Read the model definition and answer for the solid it produces. Units are mm, in the model's axes. A direction names the side the tool comes from. Coordinates: 2 decimals unless noted, no trailing zeros. Order: outer loops, then holes, each group sorted by start corner. A loop starts at its lowest first (then second) coordinate and runs counter-clockwise, first axis right, second up.
```python
from build123d import *

# Parameters (mm, degrees)
SKETCH1_W                   = 3
SKETCH1_H                   = 96
BOSS_EXTRUDE1_DEPTH         = 44.45
SKETCH2_W                   = 20
SKETCH2_H                   = 16
SKETCH2_R                   = 4
BOSS_EXTRUDE2_DEPTH         = 4
FILLET2_RADIUS              = 8
FILLET2_LENGTH              = 4
FILLET2_OF_MIRROR2_2_RADIUS = 8
FILLET2_OF_MIRROR2_2_LENGTH = 4


with BuildPart() as part:
    # Sketch1 → Boss-Extrude1 (new body)
    with BuildSketch(Plane.XY):
        Rectangle(SKETCH1_W, SKETCH1_H)
    extrude(amount=BOSS_EXTRUDE1_DEPTH)

    # Sketch2 → Boss-Extrude2 (add)
    with BuildSketch(Plane.XY.offset(44.45)):
        with Locations((11.5, -40)):
            Rectangle(SKETCH2_W, SKETCH2_H)
        with Locations((15.5, -40)):
            Circle(SKETCH2_R, mode=Mode.SUBTRACT)
    boss_extrude2 = extrude(amount=-BOSS_EXTRUDE2_DEPTH)

    # Fillet2: full round fillet: the end face becomes a half cylinder, R = half its width
    fillet2_face = Plane((21.5, -40, 42.45), x_dir=(0, 0, -1), z_dir=(1, 0, 0))  # on the end face: x along it, z out of the body
    fillet2_slab = fillet2_face.offset(-FILLET2_RADIUS / 2) * Box(FILLET2_LENGTH, 2 * FILLET2_RADIUS, FILLET2_RADIUS, mode=Mode.PRIVATE)  # the body's end, R deep
    fillet2_round = Plane((13.5, -40, 42.45), x_dir=(1, 0, 0), z_dir=(0, 0, -1)) * Cylinder(FILLET2_RADIUS, FILLET2_LENGTH, mode=Mode.PRIVATE)  # its axis R under the face
    add(fillet2_slab - fillet2_round, mode=Mode.SUBTRACT)

    # Mirror2: Boss-Extrude2 across plane
    add(boss_extrude2.mirror(Plane.XY.offset(22.225)))

    # Fillet2 of Mirror2 2: full round fillet: the end face becomes a half cylinder, R = half its width
    fillet2_of_mirror2_2_face = Plane((21.5, -40, 2), x_dir=(0, 0, 1), z_dir=(1, 0, 0))  # on the end face: x along it, z out of the body
    fillet2_of_mirror2_2_slab = fillet2_of_mirror2_2_face.offset(-FILLET2_OF_MIRROR2_2_RADIUS / 2) * Box(FILLET2_OF_MIRROR2_2_LENGTH, 2 * FILLET2_OF_MIRROR2_2_RADIUS, FILLET2_OF_MIRROR2_2_RADIUS, mode=Mode.PRIVATE)  # the body's end, R deep
    fillet2_of_mirror2_2_round = Plane((13.5, -40, 2), x_dir=(1, 0, 0), z_dir=(0, 0, 1)) * Cylinder(FILLET2_OF_MIRROR2_2_RADIUS, FILLET2_OF_MIRROR2_2_LENGTH, mode=Mode.PRIVATE)  # its axis R under the face
    add(fillet2_of_mirror2_2_slab - fillet2_of_mirror2_2_round, mode=Mode.SUBTRACT)


solid = part.part
```
1) A cutting plane is placed at C-C, the plane x = 15. Determine the outline of the cut face in (y, z), and give its area (3 significant figures).
A:
outline: (-47.86, 0) - (-43.97, 0) - (-43.97, 4) - (-47.86, 4) - close; (-47.86, 40.45) - (-43.97, 40.45) - (-43.97, 44.45) - (-47.86, 44.45) - close; (-36.03, 0) - (-32.14, 0) - (-32.14, 4) - (-36.03, 4) - close; (-36.03, 40.45) - (-32.14, 40.45) - (-32.14, 44.45) - (-36.03, 44.45) - close
area: 62.2 mm2
2) Flat-ended cylindrical pins translate along their axes: pin 1 Ø13.5 at (y, z) = (-23.5, 17) entering from +X; pin 2 Ø13 at (x, y) = (15.5, -40) entering from +Z; pin 3 Ø4.5 at (x, z) = (5, 42) entering from +Y. Find the tip coordinate at first contact, or state that the pin passes through.
A:
pin 1: stops at x = 1.5
pin 2: stops at z = 44.45
pin 3: stops at y = -32
3) Determine the mould class of faces 4 (the cylindrical face through (21.498, -39.824, 42.422)), 5 (the flat face through (7, -32, 42)), 6 (the flat face through (1, -18, 44.45)), 7 (the cylindrical face through (14.979, -36.034, 42.478)) for opening direction Y: pulls with the +Y half, pulls with the -Y half, needs draft (parallel to the pull), parting line crosses it, or undercut.
A:
face 4: parting line crosses it
face 5: pulls with the +Y half
face 6: needs draft
face 7: undercut
4) A cutting plane is placed at A-A, the plane x = 2.75. Determine the outline of the cut face in (y, z), and give its area (3 significant figures).
A:
outline: (-48, 0) - (-32, 0) - (-32, 4) - (-48, 4) - close; (-48, 40.45) - (-32, 40.45) - (-32, 44.45) - (-48, 44.45) - close
area: 128 mm2
5) A cutting plane is placed at B-B, the plane y = -40. Determine the outline of the cut face in (x, z).
A:
outline: (-1.5, 0) - (11.5, 0) - (11.5, 4) - (1.5, 4) - (1.5, 40.45) - (11.5, 40.45) - (11.5, 44.45) - (-1.5, 44.45) - close; (19.5, 0) - (21.5, 0) - (21.5, 4) - (19.5, 4) - close; (19.5, 40.45) - (21.5, 40.45) - (21.5, 44.45) - (19.5, 44.45) - close
6) A cutting plane is placed at D-D, the plane z = 13. Determine the outline of the cut face in (x, y), and give its area (3 significant figures).
A:
outline: (-1.5, -48) - (1.5, -48) - (1.5, 48) - (-1.5, 48) - close
area: 288 mm2
7) Straight lines are drawn through the part: line 1 (Z direction, x = 10.25, y = -43); line 2 (X direction, y = 24, z = 22); line 3 (Y direction, x = 15.5, z = 2.8). For each, find the intervals that lie inside material, in ascending order.
A:
line 1: z = 0 to 4, 40.45 to 44.45
line 2: x = -1.5 to 1.5
line 3: y = -47.75 to -44, -36 to -32.25
8) Which of the six approach directions +Z, -Z, +X, -X, +Y, -Y give full straight-line access (tool end or side, diameter ignored) to faces 1 (the flat face through (7, -32, 2)), 2 (the flat face through (9, -40, 40.45)), 3 (the flat face through (1, -18, 0))?
A:
face 1: +Z, -Z, +X, +Y
face 2: +X, +Y, -Y
face 3: -Z, +X, -X, +Y, -Y
